```python
from build123d import *

# Parameters (mm, degrees)
SKETCH1_R           = 75
BOSS_EXTRUDE1_DEPTH = 5
SKETCH2_R           = 60
SKETCH2_R_2         = 59
CUT_EXTRUDE1_DEPTH  = 1
SKETCH3_R           = 5
CUT_EXTRUDE2_DEPTH  = 161
CIRPATTERN2_COUNT   = 6
SKETCH4_R           = 6
CUT_EXTRUDE3_DEPTH  = 10


with BuildPart() as part:
    # Sketch1 → Boss-Extrude1 (new body)
    with BuildSketch(Plane(origin=(0, 0, 0), x_dir=(1, 0, 0), z_dir=(0, 1, 0))):
        with Locations(Location((0, 0, 0), (0, 0, 270))):
            Circle(SKETCH1_R)
    extrude(amount=BOSS_EXTRUDE1_DEPTH)

    # Sketch2 → Cut-Extrude1 (cut)
    with BuildSketch(Plane(origin=(0, 5, 0), x_dir=(1, 0, 0), z_dir=(0, 1, 0))):
        with Locations(Location((0, 0, 0), (0, 0, 270))):
            Circle(SKETCH2_R)
        with Locations(Location((0, 0, 0), (0, 0, 270))):
            Circle(SKETCH2_R_2, mode=Mode.SUBTRACT)
    extrude(amount=-CUT_EXTRUDE1_DEPTH, mode=Mode.SUBTRACT)

    # Sketch3 → Cut-Extrude2 (cut)
    with BuildSketch(Plane(origin=(0, 5, 0), x_dir=(1, 0, 0), z_dir=(0, 1, 0))):
        with Locations(Location((-67.167126111, 0, 0), (0, 0, 270))):
            Circle(SKETCH3_R)
    cut_extrude2 = extrude(amount=-CUT_EXTRUDE2_DEPTH, mode=Mode.SUBTRACT)

    # CirPattern2: Cut-Extrude2 ×6 about axis
    cirpattern2_axis = Axis((0, 0, 0), (0, 1, 0))
    for i in range(1, CIRPATTERN2_COUNT):
        add(cut_extrude2.rotate(cirpattern2_axis, i * 360 / CIRPATTERN2_COUNT), mode=Mode.SUBTRACT)

    # Sketch4 → Cut-Extrude3 (cut)
    with BuildSketch(Plane(origin=(0, 5, 0), x_dir=(1, 0, 0), z_dir=(0, 1, 0))):
        with Locations(Location((0, 0, 0), (0, 0, 270))):
            Circle(SKETCH4_R)
    extrude(amount=-CUT_EXTRUDE3_DEPTH, mode=Mode.SUBTRACT)


solid = part.part
```
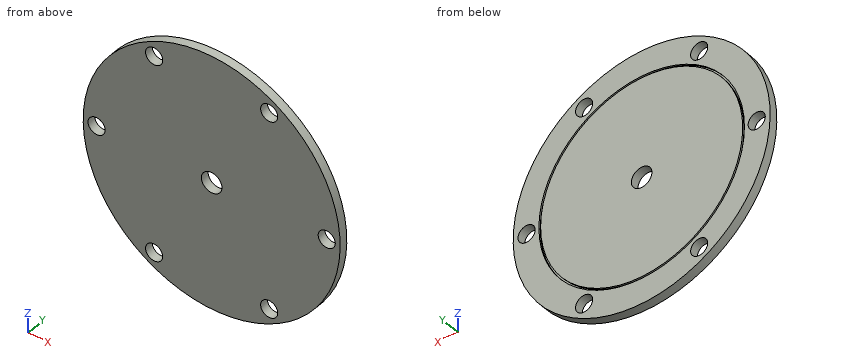
Model file for the job. Use its own axes, mm. Give positions to 0.01 mm unless a question says otherwise; leave off trailing zeros. Write each loop counter-clockwise with the first axis right and the second up, starting at its lowest first coordinate (ties: lowest second). Pieces come first, ordered by that corner, then holes. Notation, with made-up numbers: (-4.75, -13.5) -> (27.25, -13.5) arc R24 ccw to (27.25, 0.5) -> close; hole circle Ø7 at (29, 21). An arc over 180 degrees is marked (long way). Use CSV: the item, a comma, the result in double quotes. Start each with the question number.
1) Cut at B-B on x = -32. List the corners of the cut face in (y, z), plus the area to 3 significant figures.
2) Cut at C-C on x = 0. List the corners of the cut face in (y, z), plus the area to 3 significant figures.
3) Cut at A-A on z = 0. List the corners of the cut face in (x, y).
4) Pin check, flat tips, straight feed: P1, Ø3, axis at y = 3, z = 19.5, coming from the -X side; P2, Ø2, axis at x = 5.5, y = 4.5, coming from the -Z side; P3, Ø1.5, axis at y = 0.5, z = 52.5, coming from the +X side. Stop position of each tip, or through.
5) Drill centre lines: L1, parallel to Z at x = -29.5, y = 2.4; L2, parallel to X at y = 4.3, z = 1.5 (3 decimals); L3, parallel to Z at x = -3, y = 4.1. Where is each one in solid material? Low to high.
6) Cut at D-D on y = 2.8. List the corners of the cut face in (x, z).
Final values:
1,outline,"(0, -67.83) -> (5, -67.83) -> (5, -62.91) -> (0, -62.91) -> close; (0, -53.43) -> (5, -53.43) -> (5, -50.75) -> (4, -50.75) -> (4, -49.57) -> (5, -49.57) -> (5, 49.57) -> (4, 49.57) -> (4, 50.75) -> (5, 50.75) -> (5, 53.43) -> (0, 53.43) -> close; (0, 62.91) -> (5, 62.91) -> (5, 67.83) -> (0, 67.83) -> close"
1,area,"581 mm2"
2,outline,"(0, -75) -> (5, -75) -> (5, -60) -> (4, -60) -> (4, -59) -> (5, -59) -> (5, -6) -> (0, -6) -> close; (0, 6) -> (5, 6) -> (5, 59) -> (4, 59) -> (4, 60) -> (5, 60) -> (5, 75) -> (0, 75) -> close"
2,area,"688 mm2"
3,outline,"(-75, 0) -> (-72.17, 0) -> (-72.17, 5) -> (-75, 5) -> close; (-62.17, 0) -> (-6, 0) -> (-6, 5) -> (-59, 5) -> (-59, 4) -> (-60, 4) -> (-60, 5) -> (-62.17, 5) -> close; (6, 0) -> (62.17, 0) -> (62.17, 5) -> (60, 5) -> (60, 4) -> (59, 4) -> (59, 5) -> (6, 5) -> close; (72.17, 0) -> (75, 0) -> (75, 5) -> (72.17, 5) -> close"
4,P1,"stops at x = -72.81"
4,P2,"stops at z = -74.86"
4,P3,"stops at x = 54.29"
5,L1,"z = -68.95 to -61.05, -55.28 to 55.28, 61.05 to 68.95"
5,L2,"x = -74.985 to -71.937, -62.397 to -59.981, -58.981 to -5.809, 5.809 to 58.981, 59.981 to 62.397, 71.937 to 74.985"
5,L3,"z = -74.94 to -59.92, -58.92 to -5.2, 5.2 to 58.92, 59.92 to 74.94"
6,outline,"circle Ø150 at (0, 0); hole circle Ø10 at (-67.17, 0); hole circle Ø10 at (-33.58, -58.17); hole circle Ø10 at (-33.58, 58.17); hole circle Ø12 at (0, 0); hole circle Ø10 at (33.58, -58.17); hole circle Ø10 at (33.58, 58.17); hole circle Ø10 at (67.17, 0)"
